Part model, mm, in its own coordinate system. Face numbers are marked on the shaded views. A direction names the side the tool comes from. Coordinates: 2 decimals unless noted, no trailing zeros. Write each loop counter-clockwise with the first axis right and the second up, starting at its lowest first coordinate (ties: lowest second). Pieces come first, ordered by that corner, then holes. Notation, with made-up numbers: (-5, 29.5) - (8, 29.5) arc R10 cw to (8, 46.5) - close; hole circle Ø6 at (63, -27.5). An arc over 180 degrees is marked (long way). Use one line per item in the form item = value. Start each with the question number.
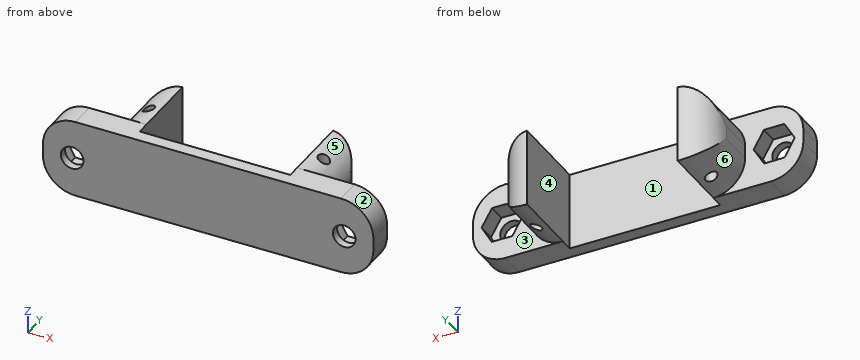
from build123d import *

# Parameters (mm, degrees)
F0_R        = 0.875
F1_DEPTH    = 12
F2_R        = 1.75
F3_DEPTH    = 25
F4_DEPTH    = 6
F5_T1_DEPTH = 36.9921862789
F5_T3_DEPTH = 22.9960931395
F5_T5_DEPTH = 29


# Not quite as in the source:
# - a fillet or chamfer that OpenCascade refuses, or shapes differently, is made with other operations: its cross-section is extruded or revolved along the edge and cut away or added


with BuildPart() as f1:
    # F0 (on Top) → F1 (new body)
    with BuildSketch(Plane.XY):
        Polygon((-11.625, -5.25), (-11.625, 7.25), (-16.5, 7.25), (-16.5, -3.25), (-16.5, -5.25), align=None)
        with Locations((-13.5, 1)):
            Circle(F0_R, mode=Mode.SUBTRACT)
        Polygon((-16.5, -5.25), (-16.5, -3.25), (-25.5, -3.25), (-25.5, -7.25), (-16.5, -7.25), align=None)
        Polygon((16.5, -3.25), (16.5, 7.25), (11.625, 7.25), (11.625, -5.25), (16.5, -5.25), align=None)
        with Locations((13.5, 1)):
            Circle(F0_R, mode=Mode.SUBTRACT)
        Polygon((25.5, -3.25), (16.5, -3.25), (16.5, -5.25), (16.5, -7.25), (25.5, -7.25), align=None)
        Polygon((16.5, -5.25), (11.625, -5.25), (-11.625, -5.25), (-16.5, -5.25), (-16.5, -7.25), (16.5, -7.25), align=None)
    extrude(amount=F1_DEPTH)

    # F2 (on Front) → F3 (cut)
    with BuildSketch(Plane.XZ):
        with Locations((21, 6)):
            Circle(F2_R)
        with Locations((-21, 6)):
            Circle(F2_R)
    extrude(amount=F3_DEPTH, mode=Mode.SUBTRACT)

    # F2 (on Front) → F4 (cut)
    with BuildSketch(Plane.XZ):
        Polygon((17.8246783439, 5.9741985751), (19.4346838614, 3.2371900682), (22.6100055175, 3.2629914931), (24.1753216561, 6.0258014249), (22.5653161386, 8.7628099318), (19.3899944825, 8.7370085069), align=None)
        with Locations((21, 6)):
            Circle(F2_R, mode=Mode.SUBTRACT)
        Polygon((-22.6100055175, 3.2629914931), (-19.4346838614, 3.2371900682), (-17.8246783439, 5.9741985751), (-19.3899944825, 8.7370085069), (-22.5653161386, 8.7628099318), (-24.1753216561, 6.0258014249), align=None)
        with Locations((-21, 6)):
            Circle(F2_R, mode=Mode.SUBTRACT)
    extrude(amount=F4_DEPTH, mode=Mode.SUBTRACT)

    # F5: fillet of radius 5 on 10 edges, made by hand

    # F5_s2 → F5_t1 (cut)
    with BuildSketch(Plane.XY.offset(-12.4960931395)):
        with BuildLine():
            ThreePointArc((-11.625, 7.25), (-15.0794552658, 5.7426227552), (-16.5, 2.2515627442))
            Line((-16.5, 2.2515627442), (-16.5, 7.25))
            Line((-16.5, 7.25), (-11.625, 7.25))
        make_face()
        with BuildLine():
            ThreePointArc((16.5, 2.2515627442), (15.0794552658, 5.7426227552), (11.625, 7.25))
            Line((11.625, 7.25), (16.5, 7.25))
            Line((16.5, 7.25), (16.5, 2.2515627442))
        make_face()
    extrude(amount=F5_T1_DEPTH, mode=Mode.SUBTRACT)

    # F5_s4 → F5_t3 (cut)
    with BuildSketch(Plane.XZ.offset(-19.7460931395)):
        with BuildLine():
            ThreePointArc((11.625, 12), (15.0794552658, 10.4926227552), (16.5, 7.0015627442))
            Line((16.5, 7.0015627442), (16.5, 12))
            Line((16.5, 12), (11.625, 12))
        make_face()
        with BuildLine():
            ThreePointArc((11.625, 0), (15.0794552658, 1.5073772448), (16.5, 4.9984372558))
            Line((16.5, 4.9984372558), (16.5, 0))
            Line((16.5, 0), (11.625, 0))
        make_face()
        with BuildLine():
            ThreePointArc((-11.625, 0), (-15.0794552658, 1.5073772448), (-16.5, 4.9984372558))
            Line((-16.5, 4.9984372558), (-16.5, 0))
            Line((-16.5, 0), (-11.625, 0))
        make_face()
        with BuildLine():
            ThreePointArc((-11.625, 12), (-15.0794552658, 10.4926227552), (-16.5, 7.0015627442))
            Line((-16.5, 7.0015627442), (-16.5, 12))
            Line((-16.5, 12), (-11.625, 12))
        make_face()
    extrude(amount=F5_T3_DEPTH, mode=Mode.SUBTRACT)

    # F5_s6 → F5_t5 (cut)
    with BuildSketch(Plane.XZ.offset(-9.25)):
        with BuildLine():
            ThreePointArc((20.5, 0), (24.0355339059, 1.4644660941), (25.5, 5))
            Line((25.5, 5), (25.5, 0))
            Line((25.5, 0), (20.5, 0))
        make_face()
        with BuildLine():
            ThreePointArc((20.5, 12), (24.0355339059, 10.5355339059), (25.5, 7))
            Line((25.5, 7), (25.5, 12))
            Line((25.5, 12), (20.5, 12))
        make_face()
        with BuildLine():
            ThreePointArc((-20.5, 12), (-24.0355339059, 10.5355339059), (-25.5, 7))
            Line((-25.5, 7), (-25.5, 12))
            Line((-25.5, 12), (-20.5, 12))
        make_face()
        with BuildLine():
            ThreePointArc((-20.5, 0), (-24.0355339059, 1.4644660941), (-25.5, 5))
            Line((-25.5, 5), (-25.5, 0))
            Line((-25.5, 0), (-20.5, 0))
        make_face()
    extrude(amount=F5_T5_DEPTH, mode=Mode.SUBTRACT)


solid = f1.part
Q1. Slice it at C-C (x = 13.5). List the corners of the cut face in (y, z) (3 decimals), plus the area to 3 significant figures.
Q2. Which spindle directions (+Z, -Z, +X, -X, +Y, -Y) get a long thin tool onto all of the face, cutting with end or side? Do the marked faces 4, 5 and 6. Say none if no direction does.
Q3. Mould opens along X. For the marked faces 1, 2 and 3 say: released by +X, released by -X, zero draft, split by the parting line, or undercut.
Q4. Slice it at D-D (y = 1). List the corners of the cut face in (x, z) (3 decimals), plus the area to 3 significant figures.
Q5. Slice it at B-B (z = 5.5). Count the separate pieces of the cut face and the enclosed holes in it, plus the area to 3 significant figures.
Q6. Drill centre lines: probe 1 along X at (y, z) = (-6.5, 6); probe 2 along X at (y, z) = (1, 6.75) (3 decimals); probe 3 along X at (y, z) = (-2, 5.5) (3 decimals). Where is each one in solid material? Low to high.
Q7. Slice it at A-A (y = -2). List the corners of the cut face in (x, z) (3 decimals).
Q8. Pin check, flat tips, straight feed: P1, Ø3.5, axis at y = 3.5, z = 5.5, coming from the +X side; P2, Ø4, axis at x = 0.5, z = 7.5, coming from the +Y side; P3, Ø1, axis at x = -14, y = 5, coming from the -Z side. Stop position of each tip, or through.
Solution:
q1.outline = (-7.25, 0) - (-3.25, 0) - (-3.25, 0.416) - (0.125, 0.416) - (0.125, 11.584) - (-3.25, 11.584) - (-3.25, 12) - (-7.25, 12) - close; (1.875, 0.416) - (6.834, 0.416) - (6.834, 11.584) - (1.875, 11.584) - close
q1.area = 141 mm2
q2.face_4 = +Z, -Z, +Y
q2.face_5 = +Z, +X, +Y
q2.face_6 = -Z, -X, +Y
q3.face_1 = undercut
q3.face_2 = released by +X
q3.face_3 = zero draft
q4.outline = (-16.5, 4.998) arc R5 ccw to (-14.375, 0.908) - (-14.375, 11.092) arc R5 ccw to (-16.5, 7.002) - close; (-12.625, 0.127) arc R5 ccw to (-11.625, 0) - (-11.625, 12) arc R5 ccw to (-12.625, 11.873) - close; (11.625, 0) arc R5 ccw to (12.625, 0.127) - (12.625, 11.873) arc R5 ccw to (11.625, 12) - close; (14.375, 0.908) arc R5 ccw to (16.5, 4.998) - (16.5, 7.002) arc R5 ccw to (14.375, 11.092) - close
q4.area = 56.7 mm2
q5.separate_pieces = 3
q5.enclosed_holes = 2
q5.area = 204 mm2
q6.probe_1 = -25.5 to -22.75, -19.25 to 19.25, 22.75 to 25.5
q6.probe_2 = -16.5 to -14.375, -12.625 to -11.625, 11.625 to 12.625, 14.375 to 16.5
q6.probe_3 = -16.5 to -11.625, 11.625 to 16.5
q7.outline = (-16.5, 4.998) arc R5 ccw to (-11.625, 0) - (-11.625, 12) arc R5 ccw to (-16.5, 7.002) - close; (11.625, 0) arc R5 ccw to (16.5, 4.998) - (16.5, 7.002) arc R5 ccw to (11.625, 12) - close
q8.P1 = 16.5
q8.P2 = -5.25
q8.P3 = 0.42
